Here's how the part is built. I have some questions about the finished solid (model axes, mm). A direction names the side the tool comes from. Give positions to 0.01 mm unless a question says otherwise; leave off trailing zeros. Loops run counter-clockwise (first coordinate to the right, second up) from the corner with the lowest first, then second, coordinate; pieces in that order, holes last.
Q1. Thinking about a two-plate mould opening in Z: for faces 1 (the face through (0.07, 0.92, -1.48)), 2 (the face through (-10.114, 1.139, -2.246)), 3 (the face through (2, 2.31, 0)), which applies, pulls with the +Z half, pulls with the -Z half, needs draft (parallel to the pull), parting line crosses it, or undercut?
Q2. I'm going to push flat-ended pins straight in: P1, Ø1.3, axis at x = 0, z = 7.125, coming from the -Y side; P2, Ø1.5, axis at x = 0, y = -2, coming from the +Z side (3 decimals); P3, Ø1.5, axis at x = -4, y = 1, coming from the -Z side; P4, Ø1.9, axis at x = -7.125, z = -3.375, coming from the -Y side. Where does each tip first touch, or does it pass through?
Q3. Suppose I cut it at D-D (z = 7.5). List the corners of the cut face in (x, y) for me.
Q4. Suppose I cut it at C-C (x = 3.75). List the corners of the cut face in (y, z) for me.
Q5. For faces 4 (the face through (-1.2, -0.43, -1.2)), 5 (the face through (-7.71, 1.17, 3.82)), which set-ups out of +Z, -Z, +X, -X, +Y, -Y let a thin tool reach every point of the face, with its end or its side?
Q6. I need wall thicknesses on probe 1 along X at (y, z) = (1.3, 0); probe 2 along Z at (x, y) = (6.75, 1.1); probe 3 along X at (y, z) = (0.55, -3.5). Which ranges of each line are inside material? Lowest first, please.
Q7. Suppose I cut it at A-A (x = 0). List the corners of the cut face in (y, z) for me (3 decimals), and give its area (3 significant figures).
Q8. Suppose I cut it at B-B (z = 0). List the corners of the cut face in (x, y) for me (3 decimals).
```python
from build123d import *

# Parameters (mm, degrees)
SKETCH1_R               = 10.36
BOSS_EXTRUDE1_DEPTH     = 2.31
BOSS_EXTRUDE2_START     = -2.31
SKETCH2_R               = 4.375
BOSS_EXTRUDE2_DEPTH     = 5.49
CUT_EXTRUDE1_DEPTH      = 16.646063403
CUT_EXTRUDE1_DEPTH_BACK = 16.646063403
SKETCH5_R               = 1.48
SKETCH6_R               = 2.79
CUT_EXTRUDE2_DEPTH      = 2.75
SKETCH7_R               = 0.735
CUT_EXTRUDE3_DEPTH      = 15.992384734
CRVPATTERN2_OUTLINE_R   = 0.735
CRVPATTERN2_DEPTH       = 2.31
CIRPATTERN1_COUNT       = 4


# Read off the part's stored shape, not the designer's step: CrvPattern2
with BuildPart() as part:
    # Sketch1 → Boss-Extrude1 (new body)
    with BuildSketch(Plane(origin=(0, 0, 0), x_dir=(1, 0, 0), z_dir=(0, 1, 0))):
        with Locations(Location((0, 0, 0), (0, 0, 270))):
            Circle(SKETCH1_R)
    extrude(amount=BOSS_EXTRUDE1_DEPTH)

    # Sketch2 → Boss-Extrude2 (add)
    with BuildSketch(Plane(origin=(0, 0, 0), x_dir=(-1, 0, 0), z_dir=(0, -1, 0)).offset(BOSS_EXTRUDE2_START)):
        with Locations(Location((0, 0, 0), (0, 0, 270))):
            Circle(SKETCH2_R)
    extrude(amount=BOSS_EXTRUDE2_DEPTH)

    # Sketch5 → Cut-Extrude1 (cut, two sides: drawn at the far end of the back side and taken through both)
    with BuildSketch(Plane(origin=(0, 2.31, 0), x_dir=(1, 0, 0), z_dir=(0, 1, 0)).offset(-CUT_EXTRUDE1_DEPTH_BACK)):
        with Locations(Location((0, 0, 0), (0, 0, 270))):
            Circle(SKETCH5_R)
    extrude(amount=CUT_EXTRUDE1_DEPTH + CUT_EXTRUDE1_DEPTH_BACK, mode=Mode.SUBTRACT)

    # Sketch6 → Cut-Extrude2 (cut)
    with BuildSketch(Plane.XZ.offset(3.18)):
        with Locations(Location((0, 0, 0), (0, 0, 270))):
            Circle(SKETCH6_R)
    extrude(amount=-CUT_EXTRUDE2_DEPTH, mode=Mode.SUBTRACT)

    # Sketch7 → Cut-Extrude3 (cut, symmetric)
    with BuildSketch(Plane(origin=(0, 0, 0), x_dir=(1, 0, 0), z_dir=(0, 1, 0))):
        with Locations(Location((-3.375, 7.125, 0), (0, 0, 270))):
            Circle(SKETCH7_R)
    cut_extrude3 = extrude(amount=CUT_EXTRUDE3_DEPTH, both=True, mode=Mode.SUBTRACT)

    # CrvPattern2 outline → CrvPattern2 (cut)
    with BuildSketch(Plane(origin=(0, 0, 0), x_dir=(1, 0, 0), z_dir=(0, 1, 0))):
        with Locations((3.375, 7.125)):
            Circle(CRVPATTERN2_OUTLINE_R)
        with Locations((0, 7.125)):
            Circle(CRVPATTERN2_OUTLINE_R)
    crvpattern2 = extrude(amount=CRVPATTERN2_DEPTH, mode=Mode.SUBTRACT)

    # CirPattern1: Cut-Extrude3, CrvPattern2 ×4 about axis
    cirpattern1_axis = Axis((0, 0, 0), (0, 1, 0))
    add([cut_extrude3.rotate(cirpattern1_axis, i * 360 / CIRPATTERN1_COUNT) for i in range(1, CIRPATTERN1_COUNT)], mode=Mode.SUBTRACT)
    add([crvpattern2.rotate(cirpattern1_axis, i * 360 / CIRPATTERN1_COUNT) for i in range(1, CIRPATTERN1_COUNT)], mode=Mode.SUBTRACT)


solid = part.part
```
Solutions:
1. face 1: undercut
1. face 2: parting line crosses it
1. face 3: needs draft
2. P1: passes through
2. P2: stops at z = 4.375
2. P3: stops at z = -9.84
2. P4: stops at y = 0
3. outline: (-7.15, 0) - (-4.01, 0) - (-4.01, 2.31) - (-7.15, 2.31) - close; (-2.74, 0) - (-0.63, 0) - (-0.63, 2.31) - (-2.74, 2.31) - close; (0.63, 0) - (2.74, 0) - (2.74, 2.31) - (0.63, 2.31) - close; (4.01, 0) - (7.15, 0) - (7.15, 2.31) - (4.01, 2.31) - close
4. outline: (-3.18, -2.25) - (0, -2.25) - (0, -6.49) - (2.31, -6.49) - (2.31, 6.49) - (0, 6.49) - (0, 2.25) - (-3.18, 2.25) - close; (0, -9.66) - (2.31, -9.66) - (2.31, -7.76) - (0, -7.76) - close; (0, 7.76) - (2.31, 7.76) - (2.31, 9.66) - (0, 9.66) - close
5. face 4: -Y
5. face 5: +Y, -Y
6. probe 1: x = -10.36 to -7.86, -6.39 to -1.48, 1.48 to 6.39, 7.86 to 10.36
6. probe 2: z = -7.86 to -4.01, -2.74 to -0.63, 0.63 to 2.74, 4.01 to 7.86
6. probe 3: x = -9.75 to -7.85, -6.4 to 6.4, 7.85 to 9.75
7. outline: (-3.18, -4.375) - (0, -4.375) - (0, -6.39) - (2.31, -6.39) - (2.31, -1.48) - (-0.43, -1.48) - (-0.43, -2.79) - (-3.18, -2.79) - close; (-3.18, 2.79) - (-0.43, 2.79) - (-0.43, 1.48) - (2.31, 1.48) - (2.31, 6.39) - (0, 6.39) - (0, 4.375) - (-3.18, 4.375) - close; (0, -10.36) - (2.31, -10.36) - (2.31, -7.86) - (0, -7.86) - close; (0, 7.86) - (2.31, 7.86) - (2.31, 10.36) - (0, 10.36) - close
7. area: 45.4 mm2
8. outline: (-10.36, 0) - (-7.86, 0) - (-7.86, 2.31) - (-10.36, 2.31) - close; (-6.39, 0) - (-4.375, 0) - (-4.375, -3.18) - (-2.79, -3.18) - (-2.79, -0.43) - (-1.48, -0.43) - (-1.48, 2.31) - (-6.39, 2.31) - close; (1.48, -0.43) - (2.79, -0.43) - (2.79, -3.18) - (4.375, -3.18) - (4.375, 0) - (6.39, 0) - (6.39, 2.31) - (1.48, 2.31) - close; (7.86, 0) - (10.36, 0) - (10.36, 2.31) - (7.86, 2.31) - close
